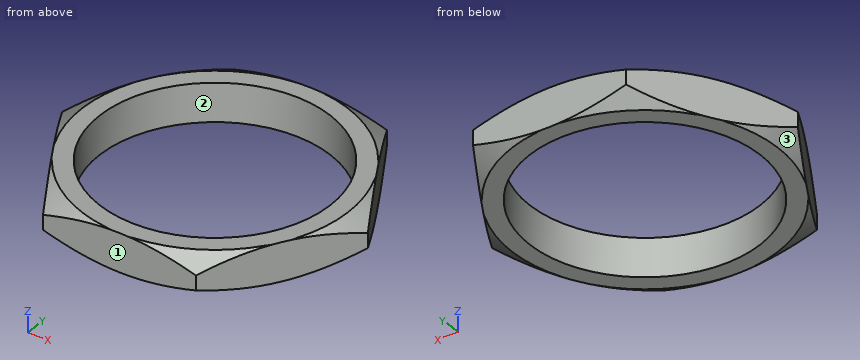
from build123d import *

# Parameters (mm, degrees)
DODANIE_WYCI_GNI_CIE1_DEPTH = 5
SZKIC2_OUTSIDE_W            = 139.232
SZKIC2_OUTSIDE_H            = 133.874
SZKIC2_OUTSIDE_R            = 17.320508076
WYTNIJ_WYCI_GNI_CIE1_DEPTH  = 25
WYTNIJ_WYCI_GNI_CIE1_DRAFT  = 60
SZKIC3_R                    = 15
WYTNIJ_WYCI_GNI_CIE5_DEPTH  = 15
SZKIC5_OUTSIDE_W            = 87.272
SZKIC5_OUTSIDE_H            = 81.914
SZKIC5_OUTSIDE_R            = 17.320508076
WYTNIJ_WYCI_GNI_CIE8_DEPTH  = 10
WYTNIJ_WYCI_GNI_CIE8_TAPER  = 60


with BuildPart() as part:
    # Szkic1 → Dodanie-wyciągnięcie1 (new body)
    with BuildSketch(Plane.XY):
        Polygon((10, 17.320508076), (-10, 17.320508076), (-20, 0), (-10, -17.320508076), (10, -17.320508076), (20, 0), align=None)
    extrude(amount=DODANIE_WYCI_GNI_CIE1_DEPTH)


with BuildPart() as wytnij_wyci_gni_cie1_tool:
    # Szkic2 outside → Wytnij-wyciągnięcie1 (with draft: the straight prism first)
    with BuildSketch(Plane.XY):
        Rectangle(SZKIC2_OUTSIDE_W, SZKIC2_OUTSIDE_H)
        Circle(SZKIC2_OUTSIDE_R, mode=Mode.SUBTRACT)
    extrude(amount=WYTNIJ_WYCI_GNI_CIE1_DEPTH)
    # Wytnij-wyciągnięcie1: the draft: its side faces are tilted about the plane it starts from
    wytnij_wyci_gni_cie1_sides = [wytnij_wyci_gni_cie1_tool.faces().sort_by_distance(p)[0] for p in [
        (0, -66.937, 12.5),
        (69.616, 0, 12.5),
        (0, 66.937, 12.5),
        (-69.616, 0, 12.5),
        (-17.320508076, 0, 12.5),
    ]]
    draft(wytnij_wyci_gni_cie1_sides, Plane.XY, WYTNIJ_WYCI_GNI_CIE1_DRAFT)


with BuildPart() as part_1:
    add(part.part)

    # Wytnij-wyciągnięcie1: cut by wytnij_wyci_gni_cie1_tool
    add(wytnij_wyci_gni_cie1_tool.part, mode=Mode.SUBTRACT)

    # Szkic3 → Wytnij-wyciągnięcie5 (cut)
    with BuildSketch(Plane.XY):
        Circle(SZKIC3_R)
    extrude(amount=WYTNIJ_WYCI_GNI_CIE5_DEPTH, mode=Mode.SUBTRACT)

    # Szkic5 outside → Wytnij-wyciągnięcie8 (cut)
    with BuildSketch(Plane.XY.offset(5)):
        Rectangle(SZKIC5_OUTSIDE_W, SZKIC5_OUTSIDE_H)
        Circle(SZKIC5_OUTSIDE_R, mode=Mode.SUBTRACT)
    extrude(amount=-WYTNIJ_WYCI_GNI_CIE8_DEPTH, taper=WYTNIJ_WYCI_GNI_CIE8_TAPER, mode=Mode.SUBTRACT)


solid = part_1.part
Source: CAD feature listing. Evaluate the final solid. Frame: model axes, mm. Face numbers are marked on the shaded views. Give positions to 0.01 mm unless a question says otherwise; leave off trailing zeros. Write item = value, one per line.
Q1. Pull-direction query (Y, two-part tool) for the marked faces 1, 2 and 3; classes: released by +Y, released by -Y, zero draft, split by the parting line, or undercut.
Data:
face_1 = released by -Y
face_2 = undercut
face_3 = split by the parting line
Q2. Material intervals for line 1 (X direction, y = 0, z = 3); line 2 (Y direction, x = -4, z = 1.1); line 3 (X direction, y = 5, z = 3.7), sorted ascending. Write a range as from..to.
Data:
line_1 = -20..-15, 15..20
line_2 = -17.32..-14.46, 14.46..17.32
line_3 = -17.11..-14.14, 14.14..17.11
Q3. Pin query (flat end, axial travel): pin 1 (1 mm diameter, centred on y = -1.5, z = 0.5, fed in from -X); pin 2 (1 mm diameter, centred on y = 2, z = 2, fed in from -X); pin 3 (1.5 mm diameter, centred on x = 12.5, z = 2, fed in from -Y). Return the tip coordinate at first contact, or that it passes through.
Data:
pin_1 = -18.99
pin_2 = -19.13
pin_3 = -14.29
